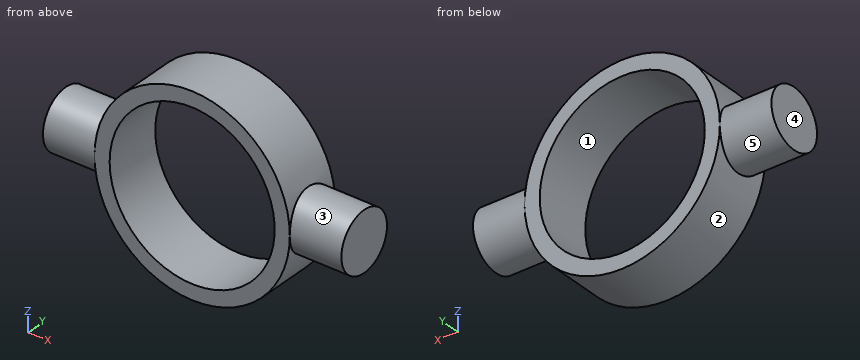
Autodesk Inventor part; units mm, degrees
ref_plane "Work Plane3" through (13.25, 8, 0) normal (1, 0, 0) x (0, 1, 0)
ref_plane "YZ Plane" through (0, 0, 0) normal (1, 0, 0) x (0, 1, 0)
ref_plane "XZ Plane" through (0, 0, 0) normal (0, 1, 0) x (-1, 0, 0)
sketch "Sketch6" plane through (0, 0, 0) normal (0, 1, 0) x (-1, 0, 0)
  circle A0 centre (0, 0) radius 4
  circle A1 centre (0, 0) radius 11.2
  circle A2 centre (0, 0) radius 14
  circle A3 centre (0, 0) radius 13.25
  line L0 (4, 13.4164) -> (-4, 13.4164)
  line L1 (19.6, 0) -> (-19.6, 0)
  point P0 (13.25, 0)
  point P1 (-13.25, 0)
  point P2 (-14, 0)
  point P3 (14, 0)
  dimension "d13" = 8
  dimension "d14" = 22.4
  dimension "d15" = 28
  dimension "d16" = 26.5
  dimension "d17" = 8
extrude "Extrusion7" add sketch "Sketch6" along normal blind 8 contours L1 A3 A1 | A1 L1 A3
sketch "Sketch9" plane through (0, 8, 0) normal (0, 1, 0) x (1, 0, 0)
  circle A0 centre (0, 0) radius 13.25
  line L0 (-18.55, 0) -> (18.55, 0)
  point P0 (13.25, 0)
ref_plane "Work Plane3" through (13.25, 8, 0) normal (1, 0, 0) x (0, 1, 0)
sketch "Sketch10" plane through (13.25, 8, 0) normal (1, 0, 0) x (0, 1, 0)
  line L0 (-9.6, 0) -> (1.6, 0)
  line L1 (-9.6, 0) -> (1.6, 0)
  line L2 (-8, 13.25) -> (0, 13.25)
  line L3 (-8, -13.25) -> (0, -13.25)
  line L4 (0, -13.25) -> (0, 13.25)
  line L5 (-8, -13.25) -> (-8, 13.25)
  line L6 (0, -13.25) -> (-8, 13.25)
  circle A0 centre (-4, 0) radius 4
  point P0 (-8, 0)
  dimension "d30" = 8
extrude "Extrusion8" add sketch "Sketch10" against normal up to surface contours A0 L6 L0 | L0 L6 A0 | L6 A0 L0 | L0 A0 L6
extrude "Extrusion9" add sketch "Sketch10" along normal blind 7 contours A0 L6 L0 | L0 L6 A0 | L6 A0 L0 | L0 A0 L6
pattern_circular "Circular Pattern3" count 2 over 360 about axis through (0, 0, 0) along (0, 1, 0) of "Extrusion8", "Extrusion9"
properties part number "anillo central"
Verification items for the finished model (mm, model axes). Face numbers are marked on the shaded views. A direction names the side the tool comes from. Coordinates: 2 decimals unless noted, no trailing zeros. Order: outer loops, then holes, each group sorted by start corner. A loop starts at its lowest first (then second) coordinate and runs counter-clockwise, first axis right, second up. Notation, with made-up numbers: (82, 19) -> (123, 19) arc R19 ccw to (123, 54) -> close; hole circle Ø11 at (44, 29). An arc over 180 degrees is marked (long way). Put each result on its own line as item: value. Start each with the question number.
1) Cross-section at C-C (z = 7.75). Enter the section's corners in (x, y), plus the area to 3 significant figures.
2) Cross-section at D-D (y = 6). Enter the section's corners in (x, z).
3) Cross-section at A-A (y = 4). Enter the section's corners in (x, z), plus the area to 3 significant figures.
4) Cross-section at B-B (x = 0). Enter the section's corners in (y, z), plus the area to 3 significant figures.
5) Go/stop test with flat-tipped pins: pin 1 (4 mm diameter, centred on x = -11.5, y = 7, fed in from -Z); pin 2 (2 mm diameter, centred on y = 4.5, z = 8, fed in from +X). Record where each tip stops, or that it passes through.
6) Material ranges on L1, parallel to Z at x = 0, y = 6.25; L2, parallel to X at y = 3, z = 0; L3, parallel to Z at x = 16.5, y = 4, recorded low to high.
7) Release check for a two-part mould opening along X. For the marked faces 1, 2 and 3 record: pulls with the +X half, pulls with the -X half, needs draft (parallel to the pull), parting line crosses it, or undercut.
8) Tool access check on the marked faces 4 and 5. Record the directions out of +Z, -Z, +X, -X, +Y, -Y that give a thin tool (end or side, any length) a straight path to the whole face; none if there is none.
Geometry check:
1. outline: (-10.75, 0) -> (-8.09, 0) -> (-8.09, 8) -> (-10.75, 8) -> close; (8.09, 0) -> (10.75, 0) -> (10.75, 8) -> (8.09, 8) -> close
1. area: 42.6 mm^2
2. outline: (-20.25, -3.46) -> (-12.79, -3.46) arc R13.25 ccw to (12.79, -3.46) -> (20.25, -3.46) -> (20.25, 3.46) -> (12.79, 3.46) arc R13.25 ccw to (-12.79, 3.46) -> (-20.25, 3.46) -> close; hole circle Ø22.4 at (0, 0)
3. outline: (-20.25, -4) -> (-12.63, -4) arc R13.25 ccw to (12.63, -4) -> (20.25, -4) -> (20.25, 4) -> (12.63, 4) arc R13.25 ccw to (-12.63, 4) -> (-20.25, 4) -> close; hole circle Ø22.4 at (0, 0)
3. area: 273 mm^2
4. outline: (0, -13.25) -> (8, -13.25) -> (8, -11.2) -> (0, -11.2) -> close; (0, 11.2) -> (8, 11.2) -> (8, 13.25) -> (0, 13.25) -> close
4. area: 32.8 mm^2
5. pin 1: stops at z = -9.24
5. pin 2: stops at x = 11.25
6. L1: z = -13.25 to -11.2, 11.2 to 13.25
6. L2: x = -20.25 to -11.2, 11.2 to 20.25
6. L3: z = -4 to 4
7. face 1: undercut
7. face 2: parting line crosses it
7. face 3: needs draft
8. face 4: +Z, -Z, -X, +Y, -Y
8. face 5: -X
